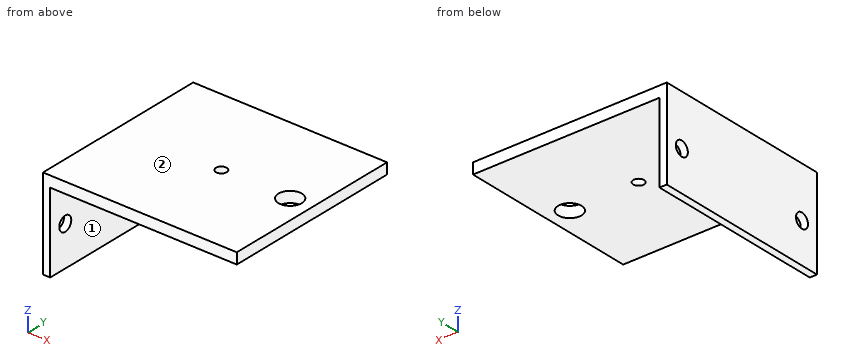
Solid Edge part; units mm, degrees
sketch "Sketch1" plane through (0, 0, 0) normal (1, 0, 0) x (0, 1, 0)
  line L0 (-50, 25) -> (-50, -25)
  line L1 (-50, -25) -> (50, -25)
  line L2 (50, -25) -> (50, 25)
  line L3 (50, 25) -> (-50, 25)
extrude "Protrusion1" add sketch "Sketch1" along normal blind 4
sketch "Sketch2" plane through (4, 0, 0) normal (1, 0, 0) x (0, 1, 0)
  line L0 (50, 19) -> (-50, 19)
  line L1 (-50, 19) -> (-50, 25)
  line L2 (-50, 25) -> (50, 25)
  line L3 (50, 25) -> (50, 19)
extrude "ExtrudedProtrusion_2" add sketch "Sketch2" along normal blind 103
sketch "Sketch3" plane through (55.5, 0, 19) normal (0, 0, -1) x (0, 1, 0)
  circle A0 centre (0, 39.5) radius 6.45
  circle A1 centre (0, 1.5) radius 3
extrude "ExtrudedCutout_1" cut sketch "Sketch3" against normal blind 28.1055
sketch "Sketch4" plane through (4, 0, 0) normal (1, 0, 0) x (0, 1, 0)
  circle A0 centre (-40, -3) radius 4
  circle A1 centre (40, -3) radius 4
extrude "Cutout1" cut sketch "Sketch4" against normal up to next
properties material "Stainless steel"
The listing builds one solid part. Answer for the finished solid, in the listing's coordinates (mm). Face numbers are marked on the shaded views. A direction names the side the tool comes from. Coordinates: 2 decimals unless noted, no trailing zeros. Order: outer loops, then holes, each group sorted by start corner. A loop starts at its lowest first (then second) coordinate and runs counter-clockwise, first axis right, second up. Notation, with made-up numbers: (72.5, -29.5) -> (88.5, -29.5) arc R28 cw to (88.5, -10.5) -> close; hole circle Ø3 at (-25.5, 74). An arc over 180 degrees is marked (long way). Answer in a Markdown table with one row per item. Add a question column.
Item 1: Find section C-C (y = 40). Write down the section's boundary in (x, z).
Item 2: Each of these flat-tipped pins is pushed along its axis until it touches: P1, Ø9, axis at y = 40, z = -3, coming from the +X side; P2, Ø2, axis at x = 16, y = 29.5, coming from the -Z side. Where does it stop, or does it pass through?
Item 3: Find section A-A (x = 57). Write down the section's boundary in (y, z).
Item 4: Which of the six approach directions +Z, -Z, +X, -X, +Y, -Y give full straight-line access (tool end or side, diameter ignored) to the marked faces 1 and 2?
Item 5: Find section D-D (x = 95). Write down the section's boundary in (y, z), then the cut area to 3 significant figures.
Item 6: Find the intervals of material crossed by L1, parallel to Z at x = 2, y = 40; L2, parallel to X at y = 0, z = 23; L3, parallel to Z at x = 91, y = -44, in increasing order. Write a range as from..to.
Item 7: Find section B-B (y = 0). Write down the section's boundary in (x, z).
Result set:
| question | item | result |
|---|---|---|
| 1 | outline | (0, -25) -> (4, -25) -> (4, -7) -> (0, -7) -> close; (0, 1) -> (4, 1) -> (4, 19) -> (107, 19) -> (107, 25) -> (0, 25) -> close |
| 2 | P1 | stops at x = 4 |
| 2 | P2 | stops at z = 19 |
| 3 | outline | (-50, 19) -> (-3, 19) -> (-3, 25) -> (-50, 25) -> close; (3, 19) -> (50, 19) -> (50, 25) -> (3, 25) -> close |
| 4 | face 1 | -Z, +X, +Y, -Y |
| 4 | face 2 | +Z, +X, -X, +Y, -Y |
| 5 | outline | (-50, 19) -> (-6.45, 19) -> (-6.45, 25) -> (-50, 25) -> close; (6.45, 19) -> (50, 19) -> (50, 25) -> (6.45, 25) -> close |
| 5 | area | 523 mm² |
| 6 | L1 | z = -25..-7, 1..25 |
| 6 | L2 | x = 0..54, 60..88.55, 101.45..107 |
| 6 | L3 | z = 19..25 |
| 7 | outline | (0, -25) -> (4, -25) -> (4, 19) -> (54, 19) -> (54, 25) -> (0, 25) -> close; (60, 19) -> (88.55, 19) -> (88.55, 25) -> (60, 25) -> close; (101.45, 19) -> (107, 19) -> (107, 25) -> (101.45, 25) -> close |
